Read the model definition and answer for the solid it produces. Units are mm, in the model's axes. Face numbers are marked on the shaded views. A direction names the side the tool comes from. Give positions to 0.01 mm unless a question says otherwise; leave off trailing zeros. Loops run counter-clockwise (first coordinate to the right, second up) from the corner with the lowest first, then second, coordinate; pieces in that order, holes last. Notation, with made-up numbers: (19, 69.5) -> (31, 69.5) arc R30 ccw to (31, 101.5) -> close; hole circle Ø5 at (15, -3). An arc over 180 degrees is marked (long way). Write each question's results on one line, items separated by ' | '. Start each with the question number.
Item 1: Which of the six approach directions +Z, -Z, +X, -X, +Y, -Y give full straight-line access (tool end or side, diameter ignored) to the marked faces 4, 5 and 6?
Item 2: Determine the mould class of the marked faces 1, 2 and 3 for opening direction Z: +Z half, -Z half, draft (parallel to the pull), parting line (faces both ways), or undercut.
Item 3: Section C-C on y = 3.5 is taken. Write down the section's boundary in (x, z), and give its area (3 significant figures).
Item 4: Section A-A on x = 0 is taken. Write down the section's boundary in (y, z), and give its area (3 significant figures).
Item 5: Each of these flat-tipped pins is pushed along its axis until it touches: P1, Ø3, axis at x = -0.5, z = -1, coming from the +Y side; P2, Ø3, axis at x = 1.5, y = 8.5, coming from the +Z side; P3, Ø5, axis at y = 23, z = 1, coming from the +X side; P4, Ø3, axis at x = 0, z = 0, coming from the +Y side. Where does it stop, or does it pass through?
Item 6: Find the intervals of material crossed by line 1 (Y direction, x = 0.5, z = 0.75); line 2 (Y direction, x = 2.5, z = 0.5); line 3 (Z direction, x = -2, y = 22.5), in increasing order.
Item 7: Section B-B on y = 17 is taken. Write down the section's boundary in (x, z), and give its area (3 significant figures).
```python
from build123d import *

# Parameters (mm, degrees)
CUT_EXTRUDE1_DEPTH = 3
FILLET1_R          = 1


with BuildPart() as part:
    # Sketch1 → Revolve1 (revolve)
    with BuildSketch(Plane.XY):
        Polygon((0, 0), (-2, 0), (-2, 6), (-3.13, 6), (-3.13, 33), (-5, 33), (-5, 37), (0, 37), align=None)
    revolve(axis=Axis((0, 37, 0), (0, -1, 0)))

    # Sketch2 → Cut-Extrude1 (cut)
    with BuildSketch(Plane(origin=(0, 37, 0), x_dir=(1, 0, 0), z_dir=(0, 1, 0))):
        Polygon((-1.154700538, -2), (1.154700538, -2), (2.309401077, 0), (1.154700538, 2), (-1.154700538, 2), (-2.309401077, 0), align=None)
    extrude(amount=-CUT_EXTRUDE1_DEPTH, mode=Mode.SUBTRACT)

    # Fillet1
    fillet1_edges = [part.edges().sort_by_distance(p)[0] for p in [
        (5, 37, 0),
    ]]
    fillet(fillet1_edges, radius=FILLET1_R)


solid = part.part
```
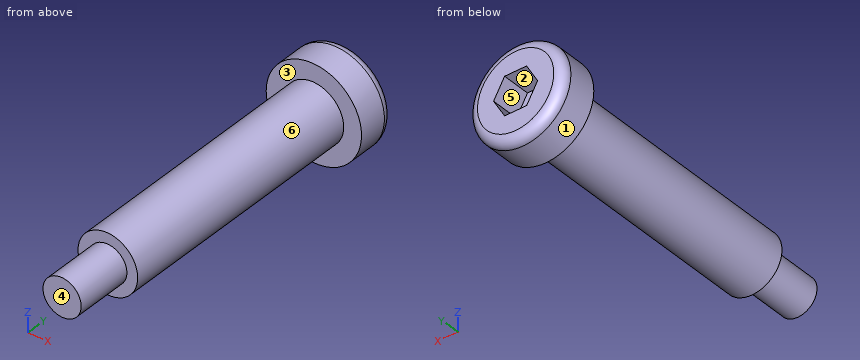
Findings:
1) face 4: +Z, -Z, +X, -X, -Y | face 5: +Y | face 6: -Y
2) face 1: parting line | face 2: undercut | face 3: draft
3) outline: circle Ø4 at (0, 0) | area: 12.6 mm2
4) outline: (0, -2) -> (6, -2) -> (6, -3.13) -> (33, -3.13) -> (33, -5) -> (36, -5) arc R1 ccw to (37, -4) -> (37, -2) -> (34, -2) -> (34, 2) -> (37, 2) -> (37, 4) arc R1 ccw to (36, 5) -> (33, 5) -> (33, 3.13) -> (6, 3.13) -> (6, 2) -> (0, 2) -> close | area: 221 mm2
5) P1: y = 37 | P2: z = 3.13 | P3: x = 3.13 | P4: y = 34
6) line 1: 0 to 34 | line 2: 6 to 37 | line 3: -2.41 to 2.41
7) outline: circle Ø6.26 at (0, 0) | area: 30.8 mm2
